from build123d import *

# Parameters (mm, degrees)
SKETCH1_R           = 1.778
BOSS_EXTRUDE1_DEPTH = 6.35
SKETCH2_W           = 19.47523672
SKETCH2_H           = 16.524840043
CUT_EXTRUDE1_DEPTH  = 10.16


with BuildPart() as part:
    # Sketch1 → Boss-Extrude1 (new body)
    with BuildSketch(Plane(origin=(0, 6.35, 0), x_dir=(1, 0, 0), z_dir=(0, 1, 0))):
        with BuildLine():
            Line((130.386666667, 6.35), (-130.386666667, 6.35))
            ThreePointArc((-130.386666667, 6.35), (-136.736666667, 0), (-130.386666667, -6.35))
            Line((-130.386666667, -6.35), (130.386666667, -6.35))
            ThreePointArc((130.386666667, -6.35), (136.736666667, 0), (130.386666667, 6.35))
        make_face()
        with Locations(Location((130.386666667, 0, 0), (0, 0, 90))):
            Circle(SKETCH1_R, mode=Mode.SUBTRACT)
        with Locations(Location((117.348, 0, 0), (0, 0, 90))):
            Circle(SKETCH1_R, mode=Mode.SUBTRACT)
        with Locations(Location((104.309333333, 0, 0), (0, 0, 90))):
            Circle(SKETCH1_R, mode=Mode.SUBTRACT)
        with Locations(Location((91.270666667, 0, 0), (0, 0, 90))):
            Circle(SKETCH1_R, mode=Mode.SUBTRACT)
        with Locations(Location((78.232, 0, 0), (0, 0, 90))):
            Circle(SKETCH1_R, mode=Mode.SUBTRACT)
        with Locations(Location((65.193333333, 0, 0), (0, 0, 90))):
            Circle(SKETCH1_R, mode=Mode.SUBTRACT)
        with Locations(Location((52.154666667, 0, 0), (0, 0, 90))):
            Circle(SKETCH1_R, mode=Mode.SUBTRACT)
        with Locations(Location((39.116, 0, 0), (0, 0, 90))):
            Circle(SKETCH1_R, mode=Mode.SUBTRACT)
        with Locations(Location((26.077333333, 0, 0), (0, 0, 90))):
            Circle(SKETCH1_R, mode=Mode.SUBTRACT)
        with Locations(Location((13.038666667, 0, 0), (0, 0, 90))):
            Circle(SKETCH1_R, mode=Mode.SUBTRACT)
        with Locations(Location((0, 0, 0), (0, 0, 90))):
            Circle(SKETCH1_R, mode=Mode.SUBTRACT)
        with Locations(Location((-13.038666667, 0, 0), (0, 0, 90))):
            Circle(SKETCH1_R, mode=Mode.SUBTRACT)
        with Locations(Location((-26.077333333, 0, 0), (0, 0, 90))):
            Circle(SKETCH1_R, mode=Mode.SUBTRACT)
        with Locations(Location((-39.116, 0, 0), (0, 0, 90))):
            Circle(SKETCH1_R, mode=Mode.SUBTRACT)
        with Locations(Location((-52.154666667, 0, 0), (0, 0, 90))):
            Circle(SKETCH1_R, mode=Mode.SUBTRACT)
        with Locations(Location((-65.193333333, 0, 0), (0, 0, 90))):
            Circle(SKETCH1_R, mode=Mode.SUBTRACT)
        with Locations(Location((-78.232, 0, 0), (0, 0, 90))):
            Circle(SKETCH1_R, mode=Mode.SUBTRACT)
        with Locations(Location((-91.270666667, 0, 0), (0, 0, 90))):
            Circle(SKETCH1_R, mode=Mode.SUBTRACT)
        with Locations(Location((-104.309333333, 0, 0), (0, 0, 90))):
            Circle(SKETCH1_R, mode=Mode.SUBTRACT)
        with Locations(Location((-117.348, 0, 0), (0, 0, 90))):
            Circle(SKETCH1_R, mode=Mode.SUBTRACT)
        with Locations(Location((-130.386666667, 0, 0), (0, 0, 90))):
            Circle(SKETCH1_R, mode=Mode.SUBTRACT)
    extrude(amount=-BOSS_EXTRUDE1_DEPTH)

    # Sketch2 → Cut-Extrude1 (cut)
    with BuildSketch(Plane(origin=(0, 6.35, 0), x_dir=(1, 0, 0), z_dir=(0, 1, 0))):
        with Locations((-133.562235071, -1.347885805)):
            Rectangle(SKETCH2_W, SKETCH2_H)
    extrude(amount=-CUT_EXTRUDE1_DEPTH, mode=Mode.SUBTRACT)


solid = part.part
Geometry check sheet. Reference: the model listing, model coordinates, mm. Give positions to 0.01 mm unless a question says otherwise; leave off trailing zeros.
1. Scan lines: line 1 (Z direction, x = 52.5, y = 5); line 2 (Z direction, x = -104, y = 1.25); line 3 (X direction, y = 4, z = 2.75). Record each from-to range of solid material in increasing order.
Completed:
line 1: z = -6.35 to -1.74, 1.74 to 6.35
line 2: z = -6.35 to -1.75, 1.75 to 6.35
line 3: x = -123.82 to 136.11
2. Sectioned sample at A-A (y = 2.75). State how many separate pieces and enclosed holes the cut face has, then the cut area to 3 significant figures.
Completed:
separate pieces: 1
enclosed holes: 20
area: 3,090 mm2
3. Depth check by flat-ended pin: pin 1 (1 mm diameter, centred on y = 1.5, z = 4.5, fed in from +X). Enter the tip coordinate at first touch or a pass-through.
Completed:
pin 1: stops at x = 135.32
